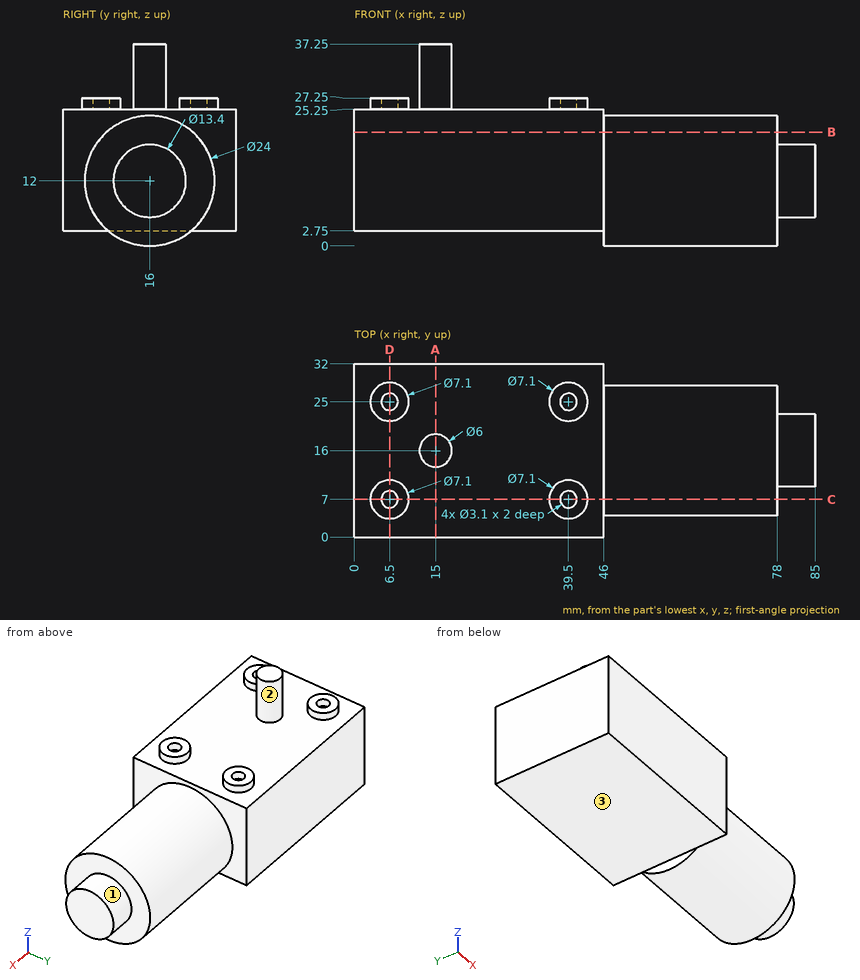
Here's the drawing with two shaded views (mm, measured from the low corner). I have some questions. A direction names the side the tool comes from. Coordinates: 2 decimals unless noted, no trailing zeros. Order: outer loops, then holes, each group sorted by start corner. A loop starts at its lowest first (then second) coordinate and runs counter-clockwise, first axis right, second up. Notation, with made-up numbers: (-27, 40) - (-3, 40) arc R25 cw to (-3, 54) - close; hole circle Ø9 at (75, -31.5). An arc over 180 degrees is marked (long way). Answer in a Markdown table with one row per item. Add a question column.
(1) If we section it at C-C, the plane y = 7: Please give me the cut outline in (x, z).
(2) On a 3-axis mill with a long thin cutter (end or side, diameter ignored), from which of +Z, -Z, +X, -X, +Y, -Y can I reach the whole of each face in a straight line? I mean the marked faces 1, 2 and 3. Say none if no direction works.
(3) If we section it at D-D, the plane x = 6.5: Please give me the cut outline in (y, z), then the cut area to 3 significant figures.
(4) If we section it at A-A, the plane x = 15: Please give me the cut outline in (y, z).
(5) If we section it at B-B, the plane z = 21: Please give me the cut outline in (x, y).
(6) Will these pins go through, and if not, where does the flat tip stop? pin 1 (8 mm diameter, centred on x = 7.5, y = 8.5, fed in from +Z); pin 2 (3.5 mm diameter, centred on x = 39.5, y = 7, fed in from -Z); pin 3 (8 mm diameter, centred on y = 6, z = 22, fed in from +X).
(7) I need wall thicknesses on L1, parallel to Y at x = 6.5, z = 25.7; L2, parallel to X at y = 25, z = 25; L3, parallel to Z at x = 21, y = 15. Which ranges of each line are inside material? Lowest first, please.
Results are:
| question | item | result |
|---|---|---|
| 1 | outline | (0, 2.75) - (46, 2.75) - (46, 4.06) - (78, 4.06) - (78, 19.94) - (46, 19.94) - (46, 25.25) - (43.05, 25.25) - (43.05, 27.25) - (41.05, 27.25) - (41.05, 25.25) - (37.95, 25.25) - (37.95, 27.25) - (35.95, 27.25) - (35.95, 25.25) - (10.05, 25.25) - (10.05, 27.25) - (8.05, 27.25) - (8.05, 25.25) - (4.95, 25.25) - (4.95, 27.25) - (2.95, 27.25) - (2.95, 25.25) - (0, 25.25) - close |
| 2 | face 1 | +X |
| 2 | face 2 | +Z |
| 2 | face 3 | -Z, -X, +Y, -Y |
| 3 | outline | (0, 2.75) - (32, 2.75) - (32, 25.25) - (28.55, 25.25) - (28.55, 27.25) - (26.55, 27.25) - (26.55, 25.25) - (23.45, 25.25) - (23.45, 27.25) - (21.45, 27.25) - (21.45, 25.25) - (10.55, 25.25) - (10.55, 27.25) - (8.55, 27.25) - (8.55, 25.25) - (5.45, 25.25) - (5.45, 27.25) - (3.45, 27.25) - (3.45, 25.25) - (0, 25.25) - close |
| 3 | area | 736 mm2 |
| 4 | outline | (0, 2.75) - (32, 2.75) - (32, 25.25) - (19, 25.25) - (19, 37.25) - (13, 37.25) - (13, 25.25) - (0, 25.25) - close |
| 5 | outline | (0, 0) - (46, 0) - (46, 8.06) - (78, 8.06) - (78, 23.94) - (46, 23.94) - (46, 32) - (0, 32) - close |
| 6 | pin 1 | stops at z = 27.25 |
| 6 | pin 2 | stops at z = 2.75 |
| 6 | pin 3 | stops at x = 78 |
| 7 | L1 | y = 3.45 to 5.45, 8.55 to 10.55, 21.45 to 23.45, 26.55 to 28.55 |
| 7 | L2 | x = 0 to 46 |
| 7 | L3 | z = 2.75 to 25.25 |
